```python
from build123d import *

# Parameters (mm, degrees)
F1_DEPTH     = 40
F2_W         = 2
F2_H         = 18
F3_DEPTH     = 18
F4_R         = 1.5875
F5_DEPTH     = 2.001
F6_R         = 1.5875
F7_DEPTH     = 2.001
F8_SIZE      = 1
F9_W         = 20
F9_H         = 18
F10_DEPTH    = 20
F12_DEPTH    = 3
F13_R        = 3.975
F14_DEPTH    = 9
F15_R        = 1
F16_R        = 9.99999
F17_R        = 3
F18_T1_DEPTH = 40.5
F19_SIZE     = 0.6


# Not quite as in the source:
# - a fillet or chamfer that OpenCascade refuses, or shapes differently, is made with other operations: its cross-section is extruded or revolved along the edge and cut away or added
# - a fillet or chamfer is up to 0.001 mm smaller than in the source, because OpenCascade refuses the exact size


with BuildPart() as f1:
    # F0 (on Front) → F1 (new body)
    with BuildSketch(Plane.XZ):
        Polygon((-2, 18), (-2, -2), (18, -2), (18, 0), (0, 0), (0, 18), align=None)
    extrude(amount=-F1_DEPTH)

    # F2 (on face) → F3 (join, through all)
    with BuildSketch(Plane.YZ):
        with Locations((1, 9)):
            Rectangle(F2_W, F2_H)
    extrude(amount=F3_DEPTH)

    # F4 (on face) → F5 (cut, through all)
    with BuildSketch(Plane.XY):
        with Locations((9, 12.5)):
            Circle(F4_R)
        with Locations((9, 27.5)):
            Circle(F4_R)
    extrude(amount=-F5_DEPTH, mode=Mode.SUBTRACT)

    # F6 (on face) → F7 (cut, through all)
    with BuildSketch(Plane.YZ):
        with Locations((35, 9)):
            Circle(F6_R)
        with Locations((20, 9)):
            Circle(F6_R)
    extrude(amount=-F7_DEPTH, mode=Mode.SUBTRACT)

    # F8
    f8_edges = [f1.edges().sort_by_distance(p)[0] for p in [
        (-2, 18.4125, 9),
        (-2, 33.4125, 9),
        (7.4125, 27.5, -2),
        (7.4125, 12.5, -2),
    ]]
    chamfer(f8_edges, length=F8_SIZE)

    # F9 (on face) → F10 (join, through all)
    with BuildSketch(Plane.XY.offset(18)):
        with Locations((8, -9)):
            Rectangle(F9_W, F9_H)
    extrude(amount=-F10_DEPTH)

    # F11 (on face) → F12 (join)
    with BuildSketch(Plane.XY.offset(18)):
        Polygon((18, -18), (18, 2), (0, 2), (-2, 2), (-2, -18), align=None)
    extrude(amount=F12_DEPTH)

    # F13 (on face) → F14 (join)
    with BuildSketch(Plane.XY.offset(21)):
        with Locations((8, -8)):
            Circle(F13_R)
    extrude(amount=F14_DEPTH)

    # F15
    f15_edges = [f1.edges().sort_by_distance(p)[0] for p in [
        (4.025, -8, 30),
    ]]
    fillet(f15_edges, radius=F15_R)

    # F16 (radius 10 in the source; OpenCascade refuses exactly that, so slightly less here)
    f16_edges = [f1.edges().sort_by_distance(p)[0] for p in [
        (-2, -18, 9.5),
        (18, -18, 9.5),
    ]]
    fillet(f16_edges, radius=F16_R)

    # F17
    f17_edges = [f1.edges().sort_by_distance(p)[0] for p in [
        (0.928929, -15.071071, 21),
        (-2, -3.000005, 21),
        (18, -3.000005, 21),
        (15.071071, -15.071071, 21),
        (8, -18, 21),
    ]]
    fillet(f17_edges, radius=F17_R)

    # F18: fillet of radius 1 on 1 edges, made by hand

    # F18_s2 → F18_t1 (cut)
    with BuildSketch(Plane.XZ.offset(-42.5)):
        with BuildLine():
            ThreePointArc((-1, 18), (-1.7071067812, 17.7071067812), (-2, 17))
            Line((-2, 17), (-2, 18))
            Line((-2, 18), (-1, 18))
        make_face()
    extrude(amount=F18_T1_DEPTH, mode=Mode.SUBTRACT)

    # F19
    f19_edges = [f1.edges().sort_by_distance(p)[0] for p in [
        (18, 15.999995, -2),
        (-2, 15.999995, -2),
        (0.928929, -15.071071, -2),
        (15.071071, -15.071071, -2),
        (8, -18, -2),
    ]]
    chamfer(f19_edges, length=F19_SIZE)


solid = f1.part
```
Source: CAD feature listing. Evaluate the final solid. Frame: model axes, mm. A direction names the side the tool comes from. Coordinates: 2 decimals unless noted, no trailing zeros. Write each loop counter-clockwise with the first axis right and the second up, starting at its lowest first coordinate (ties: lowest second). Pieces come first, ordered by that corner, then holes. Notation, with made-up numbers: (71.25, 43.25) - (109.25, 43.25) arc R12 ccw to (109.25, 52.25) - close; hole circle Ø11 at (-6.5, 5.5). An arc over 180 degrees is marked (long way). Answer as a JSON object with one key per item and string values.
Q1. Set-up query: faces 1 (the flat face through (9, 21, 0)), 2 (the cylindrical face through (4.846, -10.419, 24.944)), 3 (the flat face through (18, 1.7, 6.8)). Return all of +Z, -Z, +X, -X, +Y, -Y with unobstructed straight access to the full face (end or side cutting, diameter ignored); none if empty.
Ans:
{"face 1": "+Z, +X, +Y", "face 2": "+Z", "face 3": "+Z, -Z, +X, +Y, -Y"}
Q2. Section query B-B, the plane y = 20. Output: boundary loops of the cut face in (x, z).
Ans:
{"outline": "(-2, -1.4) - (-1.4, -2) - (17.4, -2) - (18, -1.4) - (18, 0) - (0, 0) - (0, 7.41) - (-1, 7.41) - (-2, 6.41) - close; (-2, 11.59) - (-1, 10.59) - (0, 10.59) - (0, 18) - (-1, 18) arc R1 ccw to (-2, 17) - close"}
Q3. Section query C-C, the plane y = -2.5. Output: boundary loops of the cut face in (x, z).
Ans:
{"outline": "(-2, -1.4) - (-1.4, -2) - (17.4, -2) - (18, -1.4) - (18, 18) arc R3 ccw to (15, 21) - (1, 21) arc R3 ccw to (-2, 18) - close"}
Q4. Draft query along X for faces 4 (the cylindrical face through (8.66, 25.95, -0.49)), 5 (the cylindrical face through (-1.1, -2.93, 20.14)), 6 (the flat face through (0, 21, 11)). Return one class per face: released by +X, released by -X, zero draft, split by the parting line, or undercut.
Ans:
{"face 4": "undercut", "face 5": "released by -X", "face 6": "released by +X"}
Q5. First-contact query: pin 1 Ø4 at (y, z) = (20, 7.5) entering from +X; pin 2 Ø5 at (x, z) = (1, 3.5) entering from -Y; pin 3 Ø4 at (y, z) = (-11, 1.5) entering from -X; pin 4 Ø2.5 at (x, y) = (9, 12.5) entering from +Z. Flat tips, straight axial feed; report the tip coordinate or a pass-through.
Ans:
{"pin 1": "stops at x = 0", "pin 2": "stops at y = -16.93", "pin 3": "stops at x = -1.95", "pin 4": "passes through"}
Q6. Material intervals for line 1 (Y direction, x = 9, z = -0.15); line 2 (X direction, y = 8, z = 2); line 3 (Z direction, x = -0.8, y = 35), sorted ascending. Write a range as [from, to].
Ans:
{"line 1": "y = [-17.95, 10.91], [14.09, 25.91], [29.09, 40]", "line 2": "x = [-2, 0]", "line 3": "z = [-2, 7.41], [10.59, 18]"}
Q7. Section query A-A, the plane z = 9. State how many separate pieces and enclosed holes the cut face has, plus the area to 3 significant figures.
Ans:
{"separate pieces": "3", "enclosed holes": "0", "area": "418 mm2"}
